Can you work these out from the model? Positions are in its coordinate system, mm. A direction names the side the tool comes from. Give positions to 0.01 mm unless a question says otherwise; leave off trailing zeros. Write each loop counter-clockwise with the first axis right and the second up, starting at its lowest first coordinate (ties: lowest second). Pieces come first, ordered by that corner, then holes. Notation, with made-up numbers: M 71,-15.75 L 91,-15.75 A15 ccw 91,8.25 Z; hole C 9,-38.75 d1. An arc over 180 degrees is marked long. Write each question's results on one line, items separated by ' | '.
from build123d import *

# Parameters (mm, degrees)
SKETCH1_W                                        = 46
SKETCH1_H                                        = 36
BOSS_EXTRUDE1_DEPTH                              = 4.5
SKETCH2_W                                        = 8
SKETCH2_H                                        = 7
BOSS_EXTRUDE2_DEPTH                              = 3.5
SKETCH3_W                                        = 7.999999995
SKETCH3_H                                        = 7
BOSS_EXTRUDE3_DEPTH                              = 3.5
SKETCH4_W                                        = 4
SKETCH4_H                                        = 3
F_2_05_2_05_DIAMETER_HOLE1_D                     = 2.05
F_2_05_2_05_DIAMETER_HOLE1_DEPTH                 = 8
F_2_05_2_05_DIAMETER_HOLE1_TIP                   = 0.615882135
F_2_5_2_5_DIAMETER_HOLE1_D                       = 2.5
F_2_5_2_5_DIAMETER_HOLE1_DEPTH                   = 6
F_2_5_2_5_DIAMETER_HOLE1_TIP                     = 0.751075774
CBORE_FOR_M3_HEX_HEAD_MACHINE_SCREW1_D           = 3.2
CBORE_FOR_M3_HEX_HEAD_MACHINE_SCREW1_DEPTH       = 8.000025
CBORE_FOR_M3_HEX_HEAD_MACHINE_SCREW1_CBORE_D     = 5.4
CBORE_FOR_M3_HEX_HEAD_MACHINE_SCREW1_CBORE_DEPTH = 2.5
HOLE1_D                                          = 10.4
HOLE1_CBORE_D                                    = 12.2
HOLE1_CBORE_DEPTH                                = 3.3
F_4_2_4_2_DIAMETER_HOLE1_D                       = 4.2
F_4_2_4_2_DIAMETER_HOLE1_DEPTH                   = 7
FILLET1_R                                        = 3
FILLET2_R                                        = 8


with BuildPart() as part:
    # Sketch1 → Boss-Extrude1 (new body)
    with BuildSketch(Plane.XY.offset(4.5)):
        Rectangle(SKETCH1_W, SKETCH1_H)
    extrude(amount=-BOSS_EXTRUDE1_DEPTH)

    # Sketch2 → Boss-Extrude2 (add)
    with BuildSketch(Plane.XY.offset(4.5)):
        with Locations((-19, -14.5)):
            Rectangle(SKETCH2_W, SKETCH2_H)
    extrude(amount=BOSS_EXTRUDE2_DEPTH)

    # Sketch3 → Boss-Extrude3 (add)
    with BuildSketch(Plane.XY.offset(4.5)):
        with Locations((19.000000003, -14.5)):
            Rectangle(SKETCH3_W, SKETCH3_H)
    extrude(amount=BOSS_EXTRUDE3_DEPTH)

    # Sketch4 → Revolve1 (revolve)
    with BuildSketch(Plane(origin=(0, -2, 0), x_dir=(1, 0, 0), z_dir=(0, 1, 0))):
        with Locations((-3, 1.5)):
            Rectangle(SKETCH4_W, SKETCH4_H)
    revolve(axis=Axis((-5, -2, -3), (0, 0, 1)))

    # Ø2.05 (2.05) Diameter Hole1
    with Locations(Plane(origin=(0, -18, 0), x_dir=(-1, 0, 0), z_dir=(0, -1, 0))):
        with Locations((0, -2.25)):
            Hole(F_2_05_2_05_DIAMETER_HOLE1_D / 2, depth=F_2_05_2_05_DIAMETER_HOLE1_DEPTH)
            with Locations((0, 0, -(F_2_05_2_05_DIAMETER_HOLE1_DEPTH + F_2_05_2_05_DIAMETER_HOLE1_TIP / 2))):  # 118° drill point
                Cone(0, F_2_05_2_05_DIAMETER_HOLE1_D / 2, F_2_05_2_05_DIAMETER_HOLE1_TIP, mode=Mode.SUBTRACT)

    # Ø2.5 (2.5) Diameter Hole1
    with Locations(Plane(origin=(0, -18, 0), x_dir=(-1, 0, 0), z_dir=(0, -1, 0))):
        with Locations((19, -4), (-19, -4)):
            Hole(F_2_5_2_5_DIAMETER_HOLE1_D / 2, depth=F_2_5_2_5_DIAMETER_HOLE1_DEPTH)
            with Locations((0, 0, -(F_2_5_2_5_DIAMETER_HOLE1_DEPTH + F_2_5_2_5_DIAMETER_HOLE1_TIP / 2))):  # 118° drill point
                Cone(0, F_2_5_2_5_DIAMETER_HOLE1_D / 2, F_2_5_2_5_DIAMETER_HOLE1_TIP, mode=Mode.SUBTRACT)

    # CBORE for M3 Hex Head Machine Screw1
    with Locations(Plane(origin=(0, 0, 0), x_dir=(-1, 0, 0), z_dir=(0, 0, -1))):
        with Locations((-7.962908944, 12.389389916), (10.88037403, 9.573242407), (-0.980122741, -5.337445584)):
            CounterBoreHole(CBORE_FOR_M3_HEX_HEAD_MACHINE_SCREW1_D / 2, CBORE_FOR_M3_HEX_HEAD_MACHINE_SCREW1_CBORE_D / 2, CBORE_FOR_M3_HEX_HEAD_MACHINE_SCREW1_CBORE_DEPTH, depth=CBORE_FOR_M3_HEX_HEAD_MACHINE_SCREW1_DEPTH)

    # Hole1 (through all)
    with Locations(Plane.XY.offset(4.5)):
        with Locations((-0.645780782, 5.541728913)):
            CounterBoreHole(HOLE1_D / 2, HOLE1_CBORE_D / 2, HOLE1_CBORE_DEPTH)

    # Ø4.2 (4.2) Diameter Hole1
    with Locations(Plane(origin=(0, 0, -3), x_dir=(-1, 0, 0), z_dir=(0, 0, -1))):
        with Locations((5, -2)):
            Hole(F_4_2_4_2_DIAMETER_HOLE1_D / 2, depth=F_4_2_4_2_DIAMETER_HOLE1_DEPTH)

    # Fillet1
    fillet1_edges = [part.edges().sort_by_distance(p)[0] for p in [
        (-15, -11, 6.25),
        (15.000000005, -11, 6.25),
    ]]
    fillet(fillet1_edges, radius=FILLET1_R)

    # Fillet2
    fillet2_edges = [part.edges().sort_by_distance(p)[0] for p in [
        (23, 18, 2.25),
        (-23, 18, 2.25),
    ]]
    fillet(fillet2_edges, radius=FILLET2_R)


solid = part.part
Item 1: I want a section at C-C, the plane y = -2. Please give me the cut outline in (x, z).
Geometry says:
outline: M -23,0 L -9,0 L -9,-3 L -7.1,-3 L -7.1,4 L -2.9,4 L -2.9,-3 L -1,-3 L -1,0 L 23,0 L 23,4.5 L -23,4.5 Z
Item 2: Thinking about a two-plate mould opening in X: for faces 5 (the face through (-7.133, -5.384, -1.521)), 6 (the face through (20.594, 15.719, 2.218)), 7 (the face through (1, -7.1, 2.5)), which applies, +X half, -X half, draft (parallel to the pull), parting line (faces both ways), or undercut?
Geometry says:
face 5: parting line | face 6: +X half | face 7: undercut
Item 3: I'm going to push flat-ended pins straight in: pin 1 (8.5 mm diameter, centred on x = 0.98, y = -5.34, fed in from -Z); pin 2 (4 mm diameter, centred on x = 11.5, y = -12, fed in from -Z); pin 3 (8.5 mm diameter, centred on x = 7.96, y = 12.39, fed in from +Z); pin 4 (2 mm diameter, centred on x = 19, z = 4, fed in from -Y). Where does each tip first touch, or does it pass through?
Geometry says:
pin 1: stops at z = -3 | pin 2: stops at z = 0 | pin 3: stops at z = 4.5 | pin 4: stops at y = -11.85
Item 4: For faces 1 (the face through (20, -11, 6)), 2 (the face through (-0.3, -3.7, 4.5)), 3 (the face through (-0.133, -13.944, 1.234)), 4 (the face through (2.17, 0.13, 2.87)), which set-ups out of +Z, -Z, +X, -X, +Y, -Y let a thin tool reach every point of the face, with its end or its side?
Geometry says:
face 1: +Z, +X, -X, +Y | face 2: +Z, +Y | face 3: -Y | face 4: +Z
Item 5: I want a section at A-A, the plane z = 6.5. Please give me the cut outline in (x, y).
Geometry says:
outline: M -23,-18 L -15,-18 L -15,-14 A3 ccw -18,-11 L -23,-11 Z; M 15,-18 L 23,-18 L 23,-11 L 18,-11 A3 ccw 15,-14 Z
Item 6: I want a section at D-D, the plane x = -5. Please give me the cut outline in (y, z), and give its area (3 significant figures).
Geometry says:
outline: M -18,0 L -6,0 L -6,-3 L -4.1,-3 L -4.1,4 L 0.1,4 L 0.1,-3 L 2,-3 L 2,0 L 2.7,0 L 2.7,1.2 L 1.27,1.2 L 1.27,4.5 L -18,4.5 Z; M 8.38,0 L 18,0 L 18,4.5 L 9.81,4.5 L 9.81,1.2 L 8.38,1.2 Z | area: 122 mm2
Item 7: If I drill on line 1 (X direction, y = 11, z = 0.75); line 2 (Z direction, x = 19, y = -12.5); line 3 (Z direction, x = 0, y = -12) (3 decimals), over which ranges is the centre line in solid material (lowest first)? Write a range as from..to.
Geometry says:
line 1: x = -22.94..-13.17, -8.59..5.65, 10.28..22.94 | line 2: z = 0..2.75, 5.25..8 | line 3: z = 0..1.225, 3.275..4.5
Item 8: I want a section at B-B, the plane x = -12. Please give me the cut outline in (y, z), and give its area (3 significant figures).
Geometry says:
outline: M -18,0 L 7.12,0 L 7.12,2.5 L 8.43,2.5 L 8.43,4.5 L -18,4.5 Z; M 10.72,2.5 L 12.03,2.5 L 12.03,0 L 18,0 L 18,4.5 L 10.72,4.5 Z | area: 145 mm2
